Geometry check sheet. Reference: the model listing, model coordinates, mm. A direction names the side the tool comes from. Coordinates: 2 decimals unless noted, no trailing zeros. Order: outer loops, then holes, each group sorted by start corner. A loop starts at its lowest first (then second) coordinate and runs counter-clockwise, first axis right, second up.
Autodesk Inventor part; units mm, degrees
ref_plane "Start plane" through (0, 0, 0) normal (0, 0, 1) x (1, 0, 0)
ref_plane "End plane" through (0, 0, 895.35) normal (0, 0, 1) x (1, 0, 0)
ref_plane "Work Plane3" through (0, 2.7625, 895.35) normal (0, 0, 1) x (1, 0, 0)
ref_plane "Start plane" through (0, 0, 0) normal (0, 0, 1) x (1, 0, 0)
ref_plane "End plane" through (0, 0, 895.35) normal (0, 0, 1) x (1, 0, 0)
sketch "Sketch" plane through (0, 0, 0) normal (0, 0, 1) x (1, 0, 0)
  line L0 (0, 76.2) -> (0, 0)
  line L1 (0, 0) -> (50.8, 0)
  line L2 (50.8, 0) -> (50.8, 2.7625)
  line L3 (48.8, 4.7625) -> (12.6365, 4.7625)
  line L4 (4.7625, 12.6365) -> (4.7625, 74.2)
  line L5 (2.7625, 76.2) -> (0, 76.2)
  line L6 (-7.0414, 0) -> (21.5385, 0) construction
  line L7 (0, -8.0414) -> (0, 34.5385) construction
  arc A0 (4.7625, 12.6365) -> (12.6365, 4.7625) centre (12.6365, 12.6365) ccw
  arc A1 (50.8, 2.7625) -> (48.8, 4.7625) centre (48.8, 2.7625) ccw
  arc A2 (4.7625, 74.2) -> (2.7625, 76.2) centre (2.7625, 74.2) ccw
  line L8 (0, 93.5453) -> (0, -24.9725) construction
  line L9 (-18.6925, 0) -> (62.8653, 0) construction
  point P0 (50.8, 4.7625)
  point P1 (4.7625, 4.7625)
  point P2 (4.7625, 76.2)
  dimension "d12" = 4.7625
  dimension "d13" = 76.2
  dimension "d14" = 50.8
  dimension "d15" = 0
  dimension "d16" = 4.7625
  dimension "d17" = 0
  dimension "d18" = 7.874
  dimension "d19" = 2
extrude "Body" add sketch "Sketch" along normal up to surface (895.35 mm away) from surface at 0
ref_plane "Work Plane3" through (0, 2.7625, 895.35) normal (0, 0, 1) x (1, 0, 0)
split "Split1" plane through (0, 2.7625, 895.35) removes the side toward (0, 0, 1)
equation "\"d12\" = G_T"
equation "\"d13\" = G_H"
equation "\"d14\" = G_W"
equation "\"d16\" = G_T"
equation "\"d18\" = G_IR"
equation "\"d4\" = G_L"
equation "\"G_W\" = 50.8"
equation "\"G_H\" = 76.2"
equation "\"G_T\" = 4.7625"
equation "\"G_ER\" = 4.064"
equation "\"G_IR\" = 7.874"
equation "\"G_L\" = B_L + G_OFFSET_START + G_OFFSET_END"
equation "\"ex\" = 0"
equation "\"ey\" = 0"
equation "\"G_OFFSET_START\" = 0"
equation "\"G_OFFSET_END\" = 50.8"
equation "\"d21\" = G_OFFSET_END + B_L"
equation "\"B_L\" = 844.55"
properties part number "ANSI L 3 x 2 x 3_16 00000007"
Item 1: Sectioned sample at A-A (z = 235). Record the cut outline in (x, y), and give its area (3 significant figures).
Item 2: Depth check by flat-ended pin: P1, Ø4, axis at x = 18, z = 620.5, coming from the +Y side; P2, Ø3, axis at y = 63.5, z = 485.5, coming from the +X side. Enter the tip coordinate at first touch or a pass-through.
Item 3: Tool access check on faces 1 (the face through (31, 4.762, 441)), 2 (the face through (0, 39, 441)). Record the directions out of +Z, -Z, +X, -X, +Y, -Y that give a thin tool (end or side, any length) a straight path to the whole face; none if there is none.
Item 4: Thickness scan on line 1 along X through (y, z) = (52, 220); line 2 along Y through (x, z) = (10.5, 361). Record the ranges inside material, lowest first.
Item 5: Sectioned sample at B-B (y = 57). Record the cut outline in (x, z), and give its area (3 significant figures).
Geometry check:
1. outline: (0, 0) - (50.8, 0) - (50.8, 2.76) arc R2 ccw to (48.8, 4.76) - (12.64, 4.76) arc R7.87 cw to (4.76, 12.64) - (4.76, 74.2) arc R2 ccw to (2.76, 76.2) - (0, 76.2) - close
1. area: 594 mm2
2. P1: stops at y = 4.76
2. P2: stops at x = 4.76
3. face 1: +Z, -Z, +X, +Y
3. face 2: +Z, -Z, -X, +Y, -Y
4. line 1: x = 0 to 4.76
4. line 2: y = 0 to 5.06
5. outline: (0, 0) - (4.76, 0) - (4.76, 895.35) - (0, 895.35) - close
5. area: 4,260 mm2
